Could you check a few things on this model? Use its own coordinates, in mm. A direction names the side the tool comes from. Give positions to 0.01 mm unless a question says otherwise; leave off trailing zeros. Loops run counter-clockwise (first coordinate to the right, second up) from the corner with the lowest first, then second, coordinate; pieces in that order, holes last.
1. Imagine slicing it at B-B (x = 10.5). List the corners of the cut face in (y, z) for me.
2. For faces 4 (the flat face through (9.39, 12.14, 1.588)), 5 (the cylindrical face through (9.842, 11.943, 0.783)), which set-ups out of +Z, -Z, +X, -X, +Y, -Y let a thin tool reach every point of the face, with its end or its side?
3. Imagine slicing it at A-A (y = 10). List the corners of the cut face in (x, z) for me, plus the area to 3 significant figures.
4. Thinking about a two-plate mould opening in X: for faces 1 (the flat face through (9, 1, 19.05)), 2 (the cylindrical face through (7.728, 0.783, 11.173)), 3 (the flat face through (0, 1, 5)), which applies, +X half, -X half, draft (parallel to the pull), parting line (faces both ways), or undercut?
5. Imagine slicing it at C-C (z = 9.25). List the corners of the cut face in (x, y) for me.
6. I need wall thicknesses on line 1 along Z through (x, y) = (16.75, 14.5). Which ranges of the line are inside material? Lowest first, please.
7. Imagine slicing it at D-D (x = 3.75). List the corners of the cut face in (y, z) for me, plus the area to 3 significant figures.
8. For P1, Ø6.5, axis at x = 9.525, z = 9.525, coming from the -Y side; P2, Ø4, axis at x = 9.5, y = 9.5, coming from the -Z side; P3, Ø6, axis at x = 4, y = 12.5, coming from the +Z side, each with a flat end and sliding along its axis, tell me the tip position at first contact or that it passes through.
Autodesk Inventor part; units mm, degrees
ref_plane "YZ Plane" through (0, 0, 0) normal (1, 0, 0) x (0, 1, 0)
ref_plane "XZ Plane" through (0, 0, 0) normal (0, 1, 0) x (-1, 0, 0)
ref_plane "XY Plane" through (0, 0, 0) normal (0, 0, 1) x (1, 0, 0)
sketch "Sketch1" plane through (0, 0, 0) normal (1, 0, 0) x (0, 1, 0)
  line L0 (0, 0) -> (0, 19.05)
  line L1 (0, 0) -> (19.05, 0)
  line L2 (1.5875, 19.05) -> (1.5875, 1.5875)
  line L3 (1.5875, 1.5875) -> (19.05, 1.5875)
  line L4 (0, 19.05) -> (1.5875, 19.05)
  line L5 (19.05, 0) -> (19.05, 1.5875)
  dimension "d0" = 19.05
  dimension "d1" = 19.05
  dimension "d2" = 1.5875
extrude "Extrusion1" add sketch "Sketch1" along normal blind 19.05
sketch "Sketch2" plane through (0, 0, 0) normal (0, -1, 0) x (1, 0, 0)
  line L0 (19.05, 1.5875) -> (19.05, 19.05) construction
  line L1 (19.05, 19.05) -> (0, 0) construction
  line L2 (0, 1.5875) -> (0, 19.05) construction
  line L3 (19.05, 0) -> (19.05, 1.5875) construction
  line L4 (0, 19.05) -> (19.05, 0) construction
  circle A0 centre (9.525, 9.525) radius 2.4384
  dimension "d5" = 4.8768
extrude "Extrusion2" cut sketch "Sketch2" against normal blind 25.4
sketch "Sketch3" plane through (0, 0, 0) normal (0, 0, -1) x (-1, 0, 0)
  line L0 (-19.05, 0) -> (-19.05, 19.05) construction
  line L1 (-19.05, 19.05) -> (0, 0) construction
  line L2 (0, 0) -> (0, 19.05) construction
  line L3 (0, 0) -> (-19.05, 0) construction
  line L4 (0, 19.05) -> (-19.05, 0) construction
  circle A0 centre (-9.525, 9.525) radius 2.4384
  dimension "d8" = 4.8768
extrude "Extrusion3" cut sketch "Sketch3" against normal blind 25.4
properties part number "l-bracket"
Derived:
1. outline: (0, 0) - (7.29, 0) - (7.29, 1.59) - (1.59, 1.59) - (1.59, 7.29) - (0, 7.29) - close; (0, 11.76) - (1.59, 11.76) - (1.59, 19.05) - (0, 19.05) - close; (11.76, 0) - (19.05, 0) - (19.05, 1.59) - (11.76, 1.59) - close
2. face 4: +Z, +X, -X, +Y
2. face 5: +Z, -Z
3. outline: (0, 0) - (7.13, 0) - (7.13, 1.59) - (0, 1.59) - close; (11.92, 0) - (19.05, 0) - (19.05, 1.59) - (11.92, 1.59) - close
3. area: 22.6 mm2
4. face 1: draft
4. face 2: undercut
4. face 3: -X half
5. outline: (0, 0) - (7.1, 0) - (7.1, 1.59) - (0, 1.59) - close; (11.95, 0) - (19.05, 0) - (19.05, 1.59) - (11.95, 1.59) - close
6. line 1: z = 0 to 1.59
7. outline: (0, 0) - (19.05, 0) - (19.05, 1.59) - (1.59, 1.59) - (1.59, 19.05) - (0, 19.05) - close
7. area: 58.0 mm2
8. P1: stops at y = 0
8. P2: passes through
8. P3: stops at z = 1.59
